Geometry: final body of the model. Coordinates: model frame, mm. A direction names the side the tool comes from. Coordinates: 2 decimals unless noted, no trailing zeros. Order: outer loops, then holes, each group sorted by start corner. A loop starts at its lowest first (then second) coordinate and runs counter-clockwise, first axis right, second up. Notation, with made-up numbers: M 54.5,18 L 72.5,18 A16 ccw 72.5,27 Z; hole C -12.75,54.5 d8. An arc over 180 degrees is marked long. Write item = value, one per line. Start each with the question number.
Autodesk Inventor part; units mm, degrees
ref_plane "YZ Plane" through (0, 0, 0) normal (1, 0, 0) x (0, 1, 0)
ref_plane "XZ Plane" through (0, 0, 0) normal (0, 1, 0) x (-1, 0, 0)
ref_plane "XY Plane" through (0, 0, 0) normal (0, 0, 1) x (1, 0, 0)
sketch "Sketch1" plane through (0, 0, 0) normal (0, 0, 1) x (1, 0, 0)
  circle A0 centre (0, 38.1) radius 2.1844
  circle A1 centre (0, 25.4) radius 2.1844
  circle A2 centre (0, 76.2) radius 2.1844
  circle A3 centre (0, 63.5) radius 2.1844
  line L0 (23.4735, 61.2055) -> (19.7174, 61.053)
  line L1 (17.7073, 64.2296) -> (19.7174, 61.053)
  line L2 (17.7073, 64.2296) -> (19.4532, 67.5588)
  line L3 (23.2093, 67.7113) -> (19.4532, 67.5588)
  line L4 (23.2093, 67.7113) -> (25.2195, 64.5347)
  line L5 (25.2195, 64.5347) -> (23.4735, 61.2055)
  circle A4 centre (0, 50.8) radius 7.62
  line L6 (27.0259, 61.3194) -> (5.5626, 22.3373)
  line L7 (24.5261, 69.9447) -> (3.0628, 81.7625)
  line L8 (-6.0575, 78.105) -> (-13.3265, 54.991)
  line L9 (-6.0575, 23.495) -> (-13.3265, 46.609)
  arc A5 (-6.0575, 23.495) -> (5.5626, 22.3373) centre (0, 25.4) ccw
  arc A6 (3.0628, 81.7625) -> (-6.0575, 78.105) centre (0, 76.2) ccw
  arc A7 (27.0259, 61.3194) -> (24.5261, 69.9447) centre (21.4634, 64.3821) ccw
  arc A8 (-13.3265, 54.991) -> (-13.3265, 46.609) centre (0, 50.8) ccw
  point P0 (0, 0)
  point P1 (23.4238, 61.2841)
  point P2 (10.7317, 70.2911)
  dimension "d10" = 15.24
extrude "Extrusion1" add sketch "Sketch1" along normal blind 1.524
properties part number "pto-linear-guide"
Item 1: Section query C-C on y = 77. Output: boundary loops of the cut face in (x, z) (3 decimals), and give its area (3 significant figures).
Item 2: Section query A-A on x = 0. Output: boundary loops of the cut face in (y, z).
Item 3: Section query D-D on x = 22.5. Output: boundary loops of the cut face in (y, z), and give its area (3 significant figures).
Item 4: Material intervals for probe 1 along Y at (x, z) = (0, 0.7); probe 2 along Y at (x, z) = (-1, 0.3); probe 3 along Y at (x, z) = (25, 0.5), sorted ascending. Write a range as [from, to].
Item 5: Section query B-B on z = 0.55. Give the number of separate pieces and of enclosed holes in the cut face, and give its area (3 significant figures).
Item 6: First-contact query: pin 1 (6 mm diameter, centred on x = -8.5, y = 34, fed in from -Z). Flat tip, straight axial feed; report the tip coordinate or a pass-through.
Item 7: Reachability of faces 1 (the flat face through (21.62, 61.13, 0.75)), 2 (the flat face through (-9.64, 34.89, 0.75)) from +Z, -Z, +X, -X, +Y, -Y: full face, straight path, thin tool, end or side. Return the list, or none.
Item 8: Draft query along X for faces 3 (the flat face through (7, 58, 0)), 4 (the flat face through (16.444, 42.101, 0.751)), 5 (the cylindrical face through (-0.474, 40.232, 0.751)). Return one class per face: pulls with the +X half, pulls with the -X half, needs draft (parallel to the pull), parting line crosses it, or undercut.
Ans:
q1.outline = M -6.405,0 L -2.033,0 L -2.033,1.524 L -6.405,1.524 Z; M 2.033,0 L 11.712,0 L 11.712,1.524 L 2.033,1.524 Z
q1.area = 21.4 mm^2
q2.outline = M 19.05,0 L 23.22,0 L 23.22,1.52 L 19.05,1.52 Z; M 27.58,0 L 35.92,0 L 35.92,1.52 L 27.58,1.52 Z; M 40.28,0 L 43.18,0 L 43.18,1.52 L 40.28,1.52 Z; M 58.42,0 L 61.32,0 L 61.32,1.52 L 58.42,1.52 Z; M 65.68,0 L 74.02,0 L 74.02,1.52 L 65.68,1.52 Z; M 78.38,0 L 82.55,0 L 82.55,1.52 L 78.38,1.52 Z
q3.outline = M 53.1,0 L 61.17,0 L 61.17,1.52 L 53.1,1.52 Z; M 67.68,0 L 71.06,0 L 71.06,1.52 L 67.68,1.52 Z
q3.area = 17.4 mm^2
q4.probe_1 = [19.05, 23.22], [27.58, 35.92], [40.28, 43.18], [58.42, 61.32], [65.68, 74.02], [78.38, 82.55]
q4.probe_2 = [19.13, 23.46], [27.34, 36.16], [40.04, 43.25], [58.35, 61.56], [65.44, 74.26], [78.14, 82.47]
q4.probe_3 = [57.64, 64.12], [64.88, 69.66]
q5.separate_pieces = 1
q5.enclosed_holes = 6
q5.area = 1,370 mm^2
q6.pin_1 = 0
q7.face_1 = +Z, -Z
q7.face_2 = +Z, -Z, -X, -Y
q8.face_3 = needs draft
q8.face_4 = pulls with the +X half
q8.face_5 = undercut
